Verification items for this drawing (mm, ordinates from the low corner). A direction names the side the tool comes from. Coordinates: 2 decimals unless noted, no trailing zeros. Write each loop counter-clockwise with the first axis right and the second up, starting at its lowest first coordinate (ties: lowest second). Pieces come first, ordered by that corner, then holes. Notation, with made-up numbers: (-38.75, 2.25) -> (3.25, 2.25) arc R7 cw to (3.25, 8.25) -> close; hole circle Ø11 at (80, -6). An arc over 180 degrees is marked (long way). Use CSV: the item, a comma, the result in double quotes.
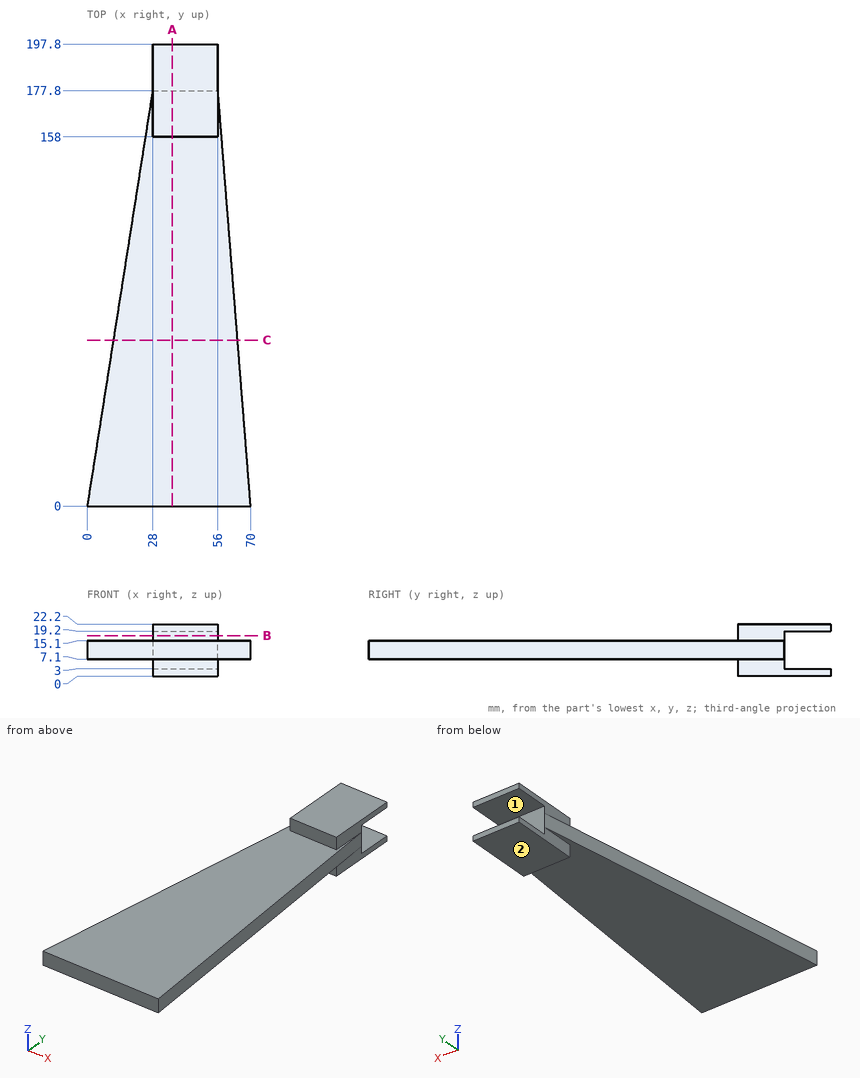
1) Scan lines: L1, parallel to Z at x = 18, y = 71; L2, parallel to Y at x = 38.5, z = 1.75; L3, parallel to Y at x = 51, z = 10.5. Record each from-to range of solid material in increasing order.
Return value:
L1,"7.1 to 15.1"
L2,"158 to 197.8"
L3,"0 to 177.8"
2) Cross-section at A-A (x = 36.5). Record the boundary of the cut face in (y, z).
Return value:
outline,"(0, 7.1) -> (158, 7.1) -> (158, 0) -> (197.8, 0) -> (197.8, 3) -> (177.8, 3) -> (177.8, 19.2) -> (197.8, 19.2) -> (197.8, 22.2) -> (158, 22.2) -> (158, 15.1) -> (0, 15.1) -> close"
3) Gauge pin test, flat ends, axial feed: pin 1 (6 mm diameter, centred on x = 25, y = 44.5, fed in from -Z); pin 2 (8 mm diameter, centred on y = 185, z = 19.5, fed in from +X); pin 3 (10 mm diameter, centred on x = 37, y = 186, fed in from -Z); pin 4 (8 mm diameter, centred on y = 185.5, z = 19.5, fed in from -X). Record the tip position at first contact, or that the pin passes through.
Return value:
pin 1,"z = 7.1"
pin 2,"x = 56"
pin 3,"z = 0"
pin 4,"x = 28"
4) Cross-section at B-B (z = 17.25). Record the boundary of the cut face in (x, y).
Return value:
outline,"(28, 158) -> (56, 158) -> (56, 177.8) -> (28, 177.8) -> close"
5) Cross-section at C-C (y = 71). Record the boundary of the cut face in (x, z), plus the area to 3 significant figures.
Return value:
outline,"(11.18, 7.1) -> (64.41, 7.1) -> (64.41, 15.1) -> (11.18, 15.1) -> close"
area,"426 mm2"
6) Set-up check for the marked faces 1 and 2: record each of +Z, -Z, +X, -X, +Y, -Y from which the full face is reachable in a straight line by a thin tool's end or side.
Return value:
face 1,"+X, -X, +Y"
face 2,"-Z, +X, -X, +Y, -Y"
